from build123d import *

# Parameters (mm, degrees)
ESQUISSE1_W      = 40
ESQUISSE1_H      = 15
ESQUISSE1_R      = 1.5
EXTRUSION1_DEPTH = 1.5
ESQUISSE2_R      = 1.5
EXTRUSION2_DEPTH = 1.5


with BuildPart() as part:
    # Esquisse1 → Extrusion1 (new body)
    with BuildSketch(Plane.XY):
        with Locations((-7.910187919, 3.943730074)):
            Rectangle(ESQUISSE1_W, ESQUISSE1_H)
        with Locations((-20.410187919, 3.943730074)):
            Circle(ESQUISSE1_R, mode=Mode.SUBTRACT)
        with Locations((-5.410187919, 3.943730074)):
            Circle(ESQUISSE1_R, mode=Mode.SUBTRACT)
    extrude(amount=EXTRUSION1_DEPTH)

    # Esquisse2 → Extrusion2 (cut)
    with BuildSketch(Plane.XY.offset(1.5)):
        with Locations((9.089812081, 8.443730074)):
            Circle(ESQUISSE2_R)
        with Locations((3.089812081, -0.556269926)):
            Circle(ESQUISSE2_R)
    extrude(amount=-EXTRUSION2_DEPTH, mode=Mode.SUBTRACT)


solid = part.part
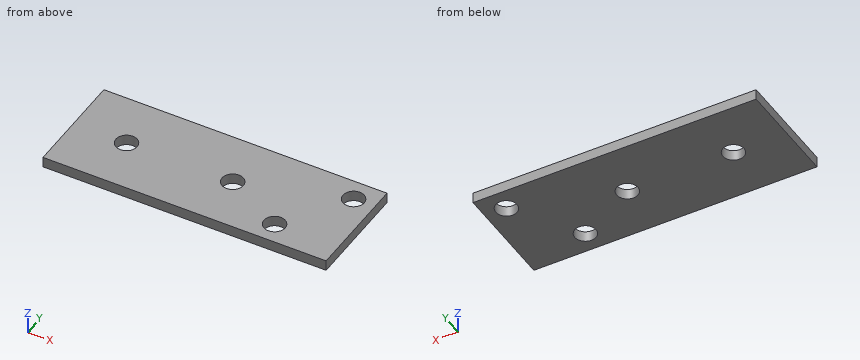
Part model, mm, in its own coordinate system. Round coordinates to 2 decimals unless told otherwise and drop trailing zeros. Order: outer loops, then holes, each group sorted by start corner. A loop starts at its lowest first (then second) coordinate and runs counter-clockwise, first axis right, second up. Notation, with made-up numbers: (8, 27) -> (34, 27) arc R16 ccw to (34, 36) -> close; hole circle Ø4 at (43, 81). An arc over 180 degrees is marked (long way). Put each result on its own line as item: value.
Q1. Band-saw the part on D-D (z = 0.85). Give the cut face in (x, y), and give its area (3 significant figures).
From the geometry:
outline: (-27.91, -3.56) -> (12.09, -3.56) -> (12.09, 11.44) -> (-27.91, 11.44) -> close; hole circle Ø3 at (-20.41, 3.94); hole circle Ø3 at (-5.41, 3.94); hole circle Ø3 at (3.09, -0.56); hole circle Ø3 at (9.09, 8.44)
area: 572 mm2
Q2. Band-saw the part on B-B (x = -19.5). Give the cut face in (y, z).
From the geometry:
outline: (-3.56, 0) -> (2.75, 0) -> (2.75, 1.5) -> (-3.56, 1.5) -> close; (5.14, 0) -> (11.44, 0) -> (11.44, 1.5) -> (5.14, 1.5) -> close
Q3. Wall check: line 1 (Y direction, x = 9, z = 0.15); line 2 (X direction, y = 3, z = 1.35); line 3 (X direction, y = 3.75, z = 0.3). Give the ranges that are in metal, low to high. Write a range as [from, to].
From the geometry:
line 1: y = [-3.56, 6.95], [9.94, 11.44]
line 2: x = [-27.91, -21.58], [-19.24, -6.58], [-4.24, 12.09]
line 3: x = [-27.91, -21.9], [-18.92, -6.9], [-3.92, 12.09]
Q4. Pin check, flat tip, straight feed: pin 1 Ø1.8 at (x, y) = (9.09, 8.44) entering from +Z. Stop position of the tip, or through.
From the geometry:
pin 1: passes through
Q5. Band-saw the part on A-A (y = 0.5). Give the cut face in (x, z).
From the geometry:
outline: (-27.91, 0) -> (2.02, 0) -> (2.02, 1.5) -> (-27.91, 1.5) -> close; (4.15, 0) -> (12.09, 0) -> (12.09, 1.5) -> (4.15, 1.5) -> close
Q6. Band-saw the part on C-C (y = 3.5). Give the cut face in (x, z).
From the geometry:
outline: (-27.91, 0) -> (-21.84, 0) -> (-21.84, 1.5) -> (-27.91, 1.5) -> close; (-18.98, 0) -> (-6.84, 0) -> (-6.84, 1.5) -> (-18.98, 1.5) -> close; (-3.98, 0) -> (12.09, 0) -> (12.09, 1.5) -> (-3.98, 1.5) -> close
